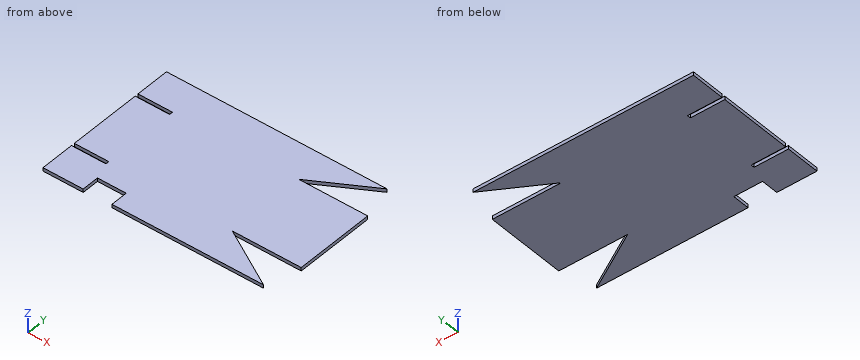
```python
from build123d import *

# Parameters (mm, degrees)
F1_DEPTH = 3


with BuildPart() as f1:
    # F0 (on Top) → F1 (new body)
    with BuildSketch(Plane.XY):
        Polygon((93.913308, 49.283788), (33.913308, 49.283788), (-76.086692, 49.283788), (-76.086692, 46.283788), (-106.086692, 46.283788), (-106.086692, -17.716212), (-76.086692, -17.716212), (-76.086692, -20.716212), (33.913308, -20.716212), (93.913308, -20.716212), align=None)
        Polygon((85.874832, -50.716212), (33.913308, -20.716212), (-76.086692, -20.716212), (-106.086692, -20.716212), (-106.086692, -50.716212), (-71.086692, -50.716212), (-71.086692, -35.716212), (-46.086692, -35.716212), (-46.086692, -50.716212), align=None)
        Polygon((85.874832, 79.283788), (-106.086692, 79.283788), (-106.086692, 49.283788), (-76.086692, 49.283788), (33.913308, 49.283788), align=None)
    extrude(amount=F1_DEPTH)


solid = f1.part
```
Read the model definition and answer for the solid it produces. Units are mm, in the model's axes. Round coordinates to 2 decimals unless told otherwise and drop trailing zeros. Write each loop counter-clockwise with the first axis right and the second up, starting at its lowest first coordinate (ties: lowest second). Pieces come first, ordered by that corner, then holes. Notation, with made-up numbers: (80.25, -10) -> (114.25, -10) arc R19 cw to (114.25, -1) -> close; hole circle Ø10 at (76, 31). An arc over 180 degrees is marked (long way). Answer in a Markdown table with one row per item. Add a question column.
1) Find section B-B, the plane x = 74. Determine the outline of the cut face in (y, z).
2) Find section A-A, the plane z = 1.1. Determine the outline of the cut face in (x, y), and give its area (3 significant figures).
3) Find section D-D, the plane x = 41. Determine the outline of the cut face in (y, z).
4) Find section C-C, the plane y = -32. Determine the outline of the cut face in (x, z).
5) Given P1, Ø0.9, axis at y = 47.5, z = 1, coming from the -X side; P2, Ø1.5, axis at x = -55.5, z = 1, coming from the -Y side, each flat-ended and moving along its own axis, determine where each tip first touches the part or whether it passes through.
6) Consider line 1 (Y direction, x = -87, z = 0.6); line 2 (Y direction, x = 51.5, z = 2.6); line 3 (Y direction, x = -68, z = 2.75). Determine where each line is inside the solid, lowest interval first.
Findings below:
| question | item | result |
|---|---|---|
| 1 | outline | (-50.72, 0) -> (-43.86, 0) -> (-43.86, 3) -> (-50.72, 3) -> close; (-20.72, 0) -> (49.28, 0) -> (49.28, 3) -> (-20.72, 3) -> close; (72.43, 0) -> (79.28, 0) -> (79.28, 3) -> (72.43, 3) -> close |
| 2 | outline | (-106.09, -50.72) -> (-71.09, -50.72) -> (-71.09, -35.72) -> (-46.09, -35.72) -> (-46.09, -50.72) -> (85.87, -50.72) -> (33.91, -20.72) -> (93.91, -20.72) -> (93.91, 49.28) -> (33.91, 49.28) -> (85.87, 79.28) -> (-106.09, 79.28) -> (-106.09, 49.28) -> (-76.09, 49.28) -> (-76.09, 46.28) -> (-106.09, 46.28) -> (-106.09, -17.72) -> (-76.09, -17.72) -> (-76.09, -20.72) -> (-106.09, -20.72) -> close |
| 2 | area | 23,400 mm² |
| 3 | outline | (-50.72, 0) -> (-24.81, 0) -> (-24.81, 3) -> (-50.72, 3) -> close; (-20.72, 0) -> (49.28, 0) -> (49.28, 3) -> (-20.72, 3) -> close; (53.38, 0) -> (79.28, 0) -> (79.28, 3) -> (53.38, 3) -> close |
| 4 | outline | (-106.09, 0) -> (53.46, 0) -> (53.46, 3) -> (-106.09, 3) -> close |
| 5 | P1 | x = -76.09 |
| 5 | P2 | y = -35.72 |
| 6 | line 1 | -50.72 to -20.72, -17.72 to 46.28, 49.28 to 79.28 |
| 6 | line 2 | -50.72 to -30.87, -20.72 to 49.28, 59.44 to 79.28 |
| 6 | line 3 | -35.72 to 79.28 |
